Source: CAD feature listing. Evaluate the final solid. Frame: model axes, mm. Face numbers are marked on the shaded views. A direction names the side the tool comes from. Coordinates: 2 decimals unless noted, no trailing zeros. Order: outer loops, then holes, each group sorted by start corner. A loop starts at its lowest first (then second) coordinate and runs counter-clockwise, first axis right, second up.
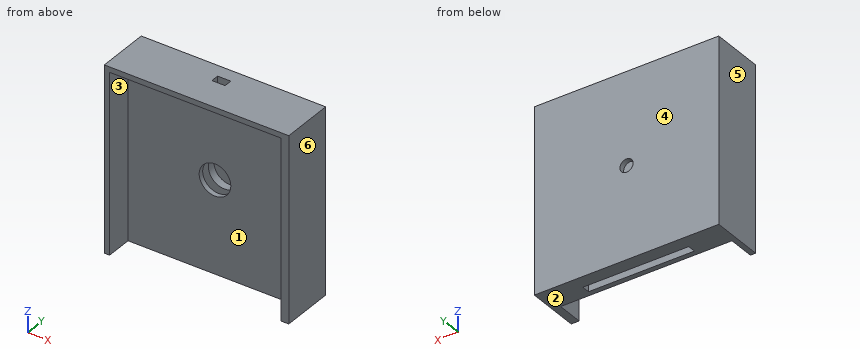
```python
from build123d import *

# Parameters (mm, degrees)
F0_W     = 70
F0_H     = 70
F0_R     = 2.5
F1_DEPTH = 20
F2_W     = 40.2
F2_H     = 3.1
F3_DEPTH = 55
F4_R     = 6
F5_DEPTH = 18
F6_W     = 65
F6_H     = 68
F7_DEPTH = 10
F8_W     = 5
F8_H     = 3.1
F9_DEPTH = 15.001


with BuildPart() as f1:
    # F0 (on Front) → F1 (new body)
    with BuildSketch(Plane.XZ):
        Rectangle(F0_W, F0_H)
        Circle(F0_R, mode=Mode.SUBTRACT)
    extrude(amount=F1_DEPTH)

    # F2 (on face) → F3 (cut)
    with BuildSketch(Plane(origin=(0, 0, -35), x_dir=(1, 0, 0), z_dir=(0, 0, -1))):
        with Locations((0, 6.55)):
            Rectangle(F2_W, F2_H)
    extrude(amount=-F3_DEPTH, mode=Mode.SUBTRACT)

    # F4 (on face) → F5 (cut)
    with BuildSketch(Plane.XZ.offset(20)):
        Circle(F4_R)
    extrude(amount=-F5_DEPTH, mode=Mode.SUBTRACT)

    # F6 (on face) → F7 (cut)
    with BuildSketch(Plane.XZ.offset(20)):
        with Locations((-0.5, -1)):
            Rectangle(F6_W, F6_H)
    extrude(amount=-F7_DEPTH, mode=Mode.SUBTRACT)

    # F8 (on face) → F9 (cut, through all)
    with BuildSketch(Plane(origin=(0, 0, 20), x_dir=(1, 0, 0), z_dir=(0, 0, -1))):
        with Locations((0, 6.55)):
            Rectangle(F8_W, F8_H)
    extrude(amount=-F9_DEPTH, mode=Mode.SUBTRACT)


solid = f1.part
```
1. Access query for the marked faces 1 and 2. Directions: +Z, -Z, +X, -X, +Y, -Y. A direction counts if a zero-diameter tool reaches every point of the face in a straight line with its end or side. Return the directions, or none.
Findings:
face 1: -Z, -Y
face 2: -Z, +X, -X, +Y, -Y
2. Draft query along X for the marked faces 3, 4, 5 and 6. Return one class per face: released by +X, released by -X, zero draft, split by the parting line, or undercut.
Findings:
face 3: undercut
face 4: zero draft
face 5: released by -X
face 6: released by +X
3. Ray query, line 1 (Y direction, x = -11.5, z = -21); line 2 (Z direction, x = 0, y = -8.9); line 3 (X direction, y = -14, z = -6). Return the intervals inside material, ascending.
Findings:
line 1: y = -10 to -8.1, -5 to 0
line 2: z = -35 to -6, 6 to 35
line 3: x = -35 to -33, 32 to 35
4. Section query B-B on x = 0. Return loops of the section in (y, z).
Findings:
outline: (-20, 33) - (-10, 33) - (-10, 6) - (-8.1, 6) - (-8.1, 35) - (-20, 35) - close; (-10, -35) - (-8.1, -35) - (-8.1, -6) - (-10, -6) - close; (-5, -35) - (0, -35) - (0, -2.5) - (-2, -2.5) - (-2, -6) - (-5, -6) - close; (-5, 6) - (-2, 6) - (-2, 2.5) - (0, 2.5) - (0, 35) - (-5, 35) - close
5. Section query D-D on z = 0. Return loops of the section in (x, y).
Findings:
outline: (-35, -20) - (-33, -20) - (-33, -10) - (-6, -10) - (-6, -8.1) - (-20.1, -8.1) - (-20.1, -5) - (-6, -5) - (-6, -2) - (-2.5, -2) - (-2.5, 0) - (-35, 0) - close; (2.5, -2) - (6, -2) - (6, -5) - (20.1, -5) - (20.1, -8.1) - (6, -8.1) - (6, -10) - (32, -10) - (32, -20) - (35, -20) - (35, 0) - (2.5, 0) - close
6. Pin query (flat end, axial travel): P1, Ø13, axis at x = -1, z = 2.5, coming from the -Y side; P2, Ø6, axis at x = -24.5, y = -14, coming from the -Z side; P3, Ø2.5, axis at x = 14.5, y = -6.5, coming from the -Z side; P4, Ø7, axis at x = 0, z = 0, coming from the +Y side. Return the tip coordinate at first contact, or that it passes through.
Findings:
P1: stops at y = -10
P2: stops at z = 33
P3: stops at z = 20
P4: stops at y = 0
7. Section query C-C on y = -9. Return loops of the section in (x, z).
Findings:
outline: (-35, -35) - (35, -35) - (35, 35) - (-35, 35) - close; hole circle Ø12 at (0, 0)
8. Section query A-A on z = 13. Return loops of the section in (x, y), plus the area to 3 significant figures.
Findings:
outline: (-35, -20) - (-33, -20) - (-33, -10) - (32, -10) - (32, -20) - (35, -20) - (35, 0) - (-35, 0) - close; hole (-20.1, -8.1) - (20.1, -8.1) - (20.1, -5) - (-20.1, -5) - close
area: 625 mm2
